```python
from build123d import *

# Parameters (mm, degrees)
SKETCH_1_W                   = 82
SKETCH_1_H                   = 20
EXTRUDE_1_DEPTH              = 8
HOLE_WIZARD_M6_1_D           = 5
HOLE_WIZARD_M6_1_CSINK_D     = 6.05
HOLE_WIZARD_M6_1_CSINK_ANGLE = 90
HOLE_WIZARD_M4_1_AT_2_COUNT  = 2
HOLE_WIZARD_M4_1_AT_2_PITCH  = 10
CHAMFER_1_SIZE               = 2


with BuildPart() as part:
    # 스케치1 → 보스-돌출1 (new body)
    with BuildSketch(Plane.XY):
        with Locations((41, 10)):
            Rectangle(SKETCH_1_W, SKETCH_1_H)
    extrude(amount=EXTRUDE_1_DEPTH)

    # M6 나사 구멍1 (through all)
    with Locations(Plane.XY.offset(8)):
        with Locations((41, 10)):
            CounterSinkHole(HOLE_WIZARD_M6_1_D / 2, HOLE_WIZARD_M6_1_CSINK_D / 2, counter_sink_angle=HOLE_WIZARD_M6_1_CSINK_ANGLE)

    # 스케치5 → M4 나사 구멍1 (revolve, cut)
    with BuildSketch(Plane(origin=(0, 15, 4), x_dir=(0, 0, 1), z_dir=(0, 1, 0))):
        Polygon((0, 0), (0, 12.491420021), (1.65, 11.5), (1.65, 0.375), (2.025, 0), align=None)
    hole_wizard_m4_1 = revolve(axis=Axis((-6.35, 15, 4), (1, 0, 0)), mode=Mode.SUBTRACT)

    # M4 나사 구멍1 at 2: M4 나사 구멍1 ×2
    with Locations(*[(0, -i * HOLE_WIZARD_M4_1_AT_2_PITCH, 0) for i in range(1, HOLE_WIZARD_M4_1_AT_2_COUNT)]):
        add(hole_wizard_m4_1, mode=Mode.SUBTRACT)

    # 대칭 복사1: M4 나사 구멍1 across plane
    add(hole_wizard_m4_1.mirror(Plane.ZY.offset(-41)), mode=Mode.SUBTRACT)

    # 대칭 복사1 copy 1 sketch → 대칭 복사1 copy 1 (revolve, cut)
    with BuildSketch(Plane(origin=(82, 5, 4), x_dir=(0, 0, 1), z_dir=(0, 1, 0))):
        Polygon((0, 0), (0, -12.491420021), (1.65, -11.5), (1.65, -0.375), (2.025, 0), align=None)
    revolve(axis=Axis((88.35, 5, 4), (1, 0, 0)), mode=Mode.SUBTRACT)

    # 모따기1
    chamfer_1_edges = [part.edges().sort_by_distance(p)[0] for p in [
        (41, 20, 8),
    ]]
    chamfer(chamfer_1_edges, length=CHAMFER_1_SIZE)


solid = part.part
```
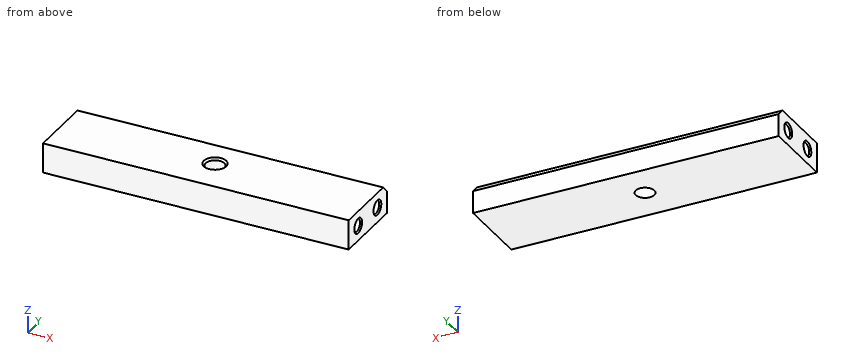
Work out the finished part from the listing and answer in its coordinate system (mm). Give positions to 0.01 mm unless a question says otherwise; leave off trailing zeros. Write each loop counter-clockwise with the first axis right and the second up, starting at its lowest first coordinate (ties: lowest second). Pieces come first, ordered by that corner, then holes.
(1) Straight lines are drawn through the part: line 1 (Y direction, x = 2.5, z = 4); line 2 (Y direction, x = 41, z = 4.5); line 3 (X direction, y = 10.25, z = 4.25). For each, find the intervals that lie inside material, in ascending order.
Final values:
line 1: y = 0 to 3.35, 6.65 to 13.35, 16.65 to 20
line 2: y = 0 to 7.5, 12.5 to 20
line 3: x = 0 to 38.51, 43.49 to 82
(2) The part is cut by section A-A on y = 10. Write down the section's boundary in (x, z) (3 decimals), plus the area to 3 significant figures.
Final values:
outline: (0, 0) - (38.5, 0) - (38.5, 7.475) - (37.975, 8) - (0, 8) - close; (43.5, 0) - (82, 0) - (82, 8) - (44.025, 8) - (43.5, 7.475) - close
area: 616 mm2
(3) A flat-ended cylindrical pin translates along its axis: pin 1 Ø2 at (y, z) = (15, 4) entering from -X. Find the tip coordinate at first contact, or state that the pin passes through.
Final values:
pin 1: stops at x = 11.89
(4) The part is cut by section B-B on x = 9. Write down the section's boundary in (y, z).
Final values:
outline: (0, 0) - (20, 0) - (20, 6) - (18, 8) - (0, 8) - close; hole circle Ø3.3 at (5, 4); hole circle Ø3.3 at (15, 4)
